```python
from build123d import *

# Parameters (mm, degrees)
SKETCH2_W           = 15.875
SKETCH2_H           = 3.175
BOSS_EXTRUDE1_DEPTH = 9.3472
CUT_EXTRUDE1_DEPTH  = 13.7
SKETCH4_R           = 1.45
BOSS_EXTRUDE2_DEPTH = 5.08


with BuildPart() as part:
    # Sketch2 → Boss-Extrude1 (new body)
    with BuildSketch(Plane(origin=(0, 0, 0), x_dir=(0, 0, -1), z_dir=(1, 0, 0))):
        with Locations((-7.9375, -1.5875)):
            Rectangle(SKETCH2_W, SKETCH2_H)
        Polygon((0, 9.525), (0, 0), (0, -3.175), (12.7, -3.175), (12.7, 9.525), align=None)
    extrude(amount=BOSS_EXTRUDE1_DEPTH)

    # Sketch3 → Cut-Extrude1 (cut, through all)
    with BuildSketch(Plane(origin=(0, 9.525, 0), x_dir=(1, 0, 0), z_dir=(0, 1, 0))):
        Polygon((3.2766, 12.7), (6.0706, 12.7), (6.1976, 3.175), (3.1496, 3.175), align=None)
    extrude(amount=-CUT_EXTRUDE1_DEPTH, mode=Mode.SUBTRACT)

    # Sketch4 → Boss-Extrude2 (add)
    with BuildSketch(Plane.XZ.offset(3.175)):
        with Locations((4.6736, 12.7)):
            Circle(SKETCH4_R)
        with Locations((4.6736, 6.35)):
            Circle(SKETCH4_R)
    extrude(amount=BOSS_EXTRUDE2_DEPTH)


solid = part.part
```
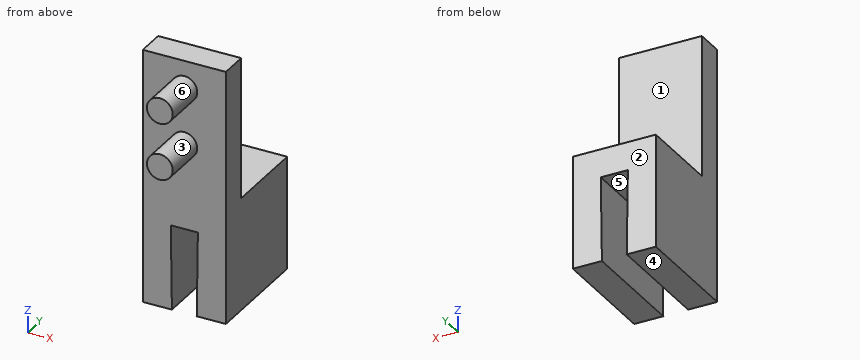
Check sheet for the modelled part. Datum: model origin and axes. Units: mm. Face numbers are marked on the shaded views. A direction names the side the tool comes from. Coordinates: 2 decimals unless noted, no trailing zeros. Order: outer loops, then holes, each group sorted by start corner. A loop starts at its lowest first (then second) coordinate and runs counter-clockwise, first axis right, second up. Notation, with made-up numbers: M 22,-12 L 40,-12 A24 cw 40,15 Z; hole C -13.5,-12.5 d5. An arc over 180 degrees is marked long. Write each question's results on one line, items separated by ' | '. Start each with the question number.
1. Cross-section at B-B on y = 5.5. Record the cut outline in (x, z) (3 decimals).
2. Cross-section at D-D on x = 2.75. Record the cut outline in (y, z) (3 decimals), and give its area (3 significant figures).
3. Go/stop test with flat-tipped pins: P1, Ø0.9, axis at x = 5, y = 1, coming from the -Z side (3 decimals); P2, Ø1, axis at x = 4, z = 5, coming from the +Y side; P3, Ø2, axis at x = 3, y = 3.5, coming from the +Z side. Record where each tip stops, or that it passes through.
4. Mould release check, pull along X, two halves, no side actions. Record for the marked faces 4, 5 and 6: +X half, -X half, draft (parallel to the pull), parting line (faces both ways), or undercut.
5. Cross-section at A-A on z = -4. Record the cut outline in (x, y) (3 decimals).
6. Access from +Z, -Z, +X, -X, +Y, -Y to the whole of each face (thin tool, end or side, straight path). Record for the marked faces 1, 2 and 3.
7. Material ranges on probe 1 along Y at (x, z) = (5.5, -1.5) (3 decimals); probe 2 along Z at (x, y) = (8.75, 8); probe 3 along Z at (x, y) = (3.5, -3) (3 decimals), recorded low to high.
8. Cross-section at C-C on z = 6.35. Record the cut outline in (x, y) (3 decimals), and give its area (3 significant figures).
Checks:
1) outline: M 0,-12.7 L 3.277,-12.7 L 3.15,-3.175 L 6.198,-3.175 L 6.071,-12.7 L 9.347,-12.7 L 9.347,0 L 0,0 Z
2) outline: M -3.175,-12.7 L 9.525,-12.7 L 9.525,0 L 0,0 L 0,15.875 L -3.175,15.875 Z | area: 212 mm²
3) P1: stops at z = -3.175 | P2: stops at y = 0 | P3: stops at z = 0
4) face 4: draft | face 5: undercut | face 6: parting line
5) outline: M 0,-3.175 L 3.161,-3.175 L 3.161,9.525 L 0,9.525 Z; M 6.187,-3.175 L 9.347,-3.175 L 9.347,9.525 L 6.187,9.525 Z
6) face 1: +Z, +X, -X, +Y | face 2: +Z, -Z, +X, -X, +Y | face 3: -Y
7) probe 1: y = -3.175 to 9.525 | probe 2: z = -12.7 to 0 | probe 3: z = -3.175 to 15.875
8) outline: M 0,-3.175 L 3.224,-3.175 L 3.224,-8.255 L 6.124,-8.255 L 6.124,-3.175 L 9.347,-3.175 L 9.347,0 L 0,0 Z | area: 44.4 mm²
